Autodesk Inventor part; units mm, degrees
ref_plane "YZ Plane" through (0, 0, 0) normal (1, 0, 0) x (0, 1, 0)
ref_plane "XZ Plane" through (0, 0, 0) normal (0, 1, 0) x (-1, 0, 0)
ref_plane "XY Plane" through (0, 0, 0) normal (0, 0, 1) x (1, 0, 0)
sketch "スケッチ1" plane through (0, 0, 0) normal (0, 0, 1) x (1, 0, 0)
  circle A0 centre (0, 0) radius 60
  dimension "d0" = 120
extrude "押し出し1" add sketch "スケッチ1" along normal blind 3
sketch "スケッチ2" plane through (0, 0, 3) normal (0, 0, 1) x (1, 0, 0)
  circle A0 centre (0, 0) radius 46
  line L0 (0, 0) -> (0, 59.211)
  line L1 (0, 0) -> (-21.8609, 52.777)
  line L2 (0, 0) -> (27.8226, 47.8581)
  point P0 (-17.6034, 42.4985)
  point P1 (-42.4985, 17.6034)
  point P2 (-42.4985, -17.6034)
  point P3 (-17.6034, -42.4985)
  point P4 (17.6034, -42.4985)
  point P5 (42.4985, -17.6034)
  point P6 (42.4985, 17.6034)
  point P7 (17.6034, 42.4985)
  dimension "d4" = 92
  dimension "d5" = 22.5
  dimension "d8" = 360
hole "穴1" at (-17.6034, 42.4985, 3) at (-42.4985, 17.6034, 3) at (-42.4985, -17.6034, 3) at (-17.6034, -42.4985, 3) at (17.6034, -42.4985, 3) at (42.4985, -17.6034, 3) at (42.4985, 17.6034, 3) at (17.6034, 42.4985, 3) direction (0, 0, -1) diameter 3.2 end through all
sketch "スケッチ4" plane through (0, 0, 0) normal (0, 0, -1) x (-1, 0, 0)
  line L0 (0, 0) -> (0, -80.557)
  circle A0 centre (0, 0) radius 60
  line L1 (-60, 0) -> (-60, -190)
  line L2 (60, 0) -> (60, -190)
  line L3 (-60, -190) -> (60, -190)
  line L4 (-60, 0) -> (-43.3772, -190)
  line L5 (10.9847, -144.6101) -> (60, -190)
  line L6 (18.2202, -151.3104) -> (-10.1159, -125.0702)
  line L7 (10, -105.557) -> (10, -25)
  circle A1 centre (0, 0) radius 7
  line L8 (10, -177.6776) -> (0, -177.6776)
  line L9 (0, -177.6776) -> (0, -62.3224)
  line L10 (10, -62.3224) -> (10, -177.6776)
  circle A2 centre (0, -160) radius 4
  circle A3 centre (0, -160) radius 15
  line L11 (27.6237, -152.2466) -> (-9.3418, -192.1645)
  line L12 (15, -160) -> (15, -138.6677)
  line L13 (30, -190) -> (10, -115.4165)
  point P0 (60, 0)
  point P1 (-59.0885, -10.4189)
  point P2 (-60, -25)
  point P3 (60, -25)
  point P4 (10, -59.1608)
  point P5 (10, -143.6982)
  point P6 (0, -134.4378)
  point P7 (0, -60)
  point P8 (0, -60)
  point P9 (10, -120)
  point P10 (10, -171.1803)
  point P11 (11.0058, -170.1918)
  point P12 (10, -171.2779)
  point P13 (21.6159, -158.7342)
  point P14 (-7.3373, -190)
  dimension "d362" = 30
  dimension "d21" = 60
  dimension "d23" = 120
  dimension "d24" = 190
  dimension "d25" = 190
  dimension "d56" = 0
  dimension "d90" = 85
  dimension "d307" = 10
  dimension "d359" = 160
  dimension "d361" = 8
  dimension "d379" = 30
  dimension "d380" = 0
  dimension "d381" = 70
extrude "押し出し3" add sketch "スケッチ4" against normal blind 3 contours L0 A0 L7 L10 L6 L9 | L0 L9 A3 L8 L11 L3 L4 A0 | L6 L10 A3 L9 | L4 L3 L1 A0 | L10 L13 L5 L6 | L6 L5 L12 A3 L10 | A3 L10 L9 A2 | L9 A2 A3 | A3 L10 | A3 L10 L11 L8 L9 | L11 L8 L10 L13 L3 | L5 L13 L11 A3 L12 | A3 L11 L10 | L11 L10 L8
sketch "スケッチ17" plane through (0, 0, 3) normal (0, 0, 1) x (1, 0, 0)
  circle A0 centre (0, 0) radius 30
  dimension "d159" = 60
extrude "押し出し10" cut sketch "スケッチ17" against normal blind 10
sketch "スケッチ20" plane through (0, 0, 3) normal (0, 0, 1) x (1, 0, 0)
  line L0 (-30, -190) -> (60, -190)
  circle A0 centre (0, 0) radius 30
  line L1 (60, -190) -> (60, 0)
  point P0 (0, -160)
  point P1 (15, -190)
  point P2 (-60, -190)
  point P3 (7.3373, -190)
  dimension "d205" = 160
  dimension "d223" = 60
  dimension "d246" = 60
hole "穴8" at (0, -160, 3) direction (0, 0, -1) diameter 8.1 end through all
fillet "フィレット4" radius 10 3 edges at (60, -190, 1.5) (-10, -115.4165, 1.5) (-30, -190, 1.5)
sketch "スケッチ28" plane through (0, 0, 3) normal (0, 0, 1) x (1, 0, 0)
  circle A0 centre (0, 0) radius 60
  circle A1 centre (0, 0) radius 54
  point P0 (0, 54)
  point P1 (-38.1838, 38.1838)
  point P2 (-54, 0)
  point P3 (-38.1838, -38.1838)
  point P4 (0, -54)
  point P5 (38.1838, -38.1838)
  point P6 (54, 0)
  point P7 (38.1838, 38.1838)
  dimension "d309" = 108
  dimension "d308" = 120
  dimension "d312" = 360
hole "穴13" at (-38.1838, -38.1838, 3) at (-54, 0, 3) at (-38.1838, 38.1838, 3) at (0, 54, 3) at (38.1838, 38.1838, 3) at (54, 0, 3) direction (0, 0, -1) diameter 3.2 end through all
sketch "スケッチ29" plane through (0, 0, 3) normal (0, 0, 1) x (1, 0, 0)
  arc A0 (60, 0) -> (-10, -59.1608) centre (0, 0) ccw
  line L0 (-10, -59.1608) -> (0, -59.1608)
  line L1 (0, -59.1608) -> (0, -130)
  line L2 (0, -130) -> (-10, -130)
  line L3 (-10, -130) -> (-10, -59.1608)
  line L4 (60, 0) -> (60, -180)
  line L5 (60, -130) -> (50, -130)
  line L6 (50, -130) -> (50, 10.2883)
  line L7 (50, 10.2883) -> (60, 10.2883)
  line L8 (60, 10.2883) -> (60, -130)
  line L9 (-30, -190) -> (50, -190)
  circle A1 centre (54, 0) radius 1.6
  line L10 (-10, -59.1608) -> (-10, -115.4165)
  point P0 (-35.8579, -190)
  point P1 (54, -40)
  point P2 (-5, -59.1608)
  point P3 (-4, -69.1608)
  point P4 (54, -80)
  point P5 (54, -120)
  point P6 (54, -160)
  point P7 (55, -130)
  point P8 (-5, -130)
  point P9 (-4, -129.1608)
  point P10 (54, -200)
  point P11 (-10, -140)
  point P12 (40, -210)
  point P13 (-40, -210)
  point P14 (-4, -99.1608)
  point P15 (7.3373, -190)
  point P16 (11.7061, -190)
  dimension "d321" = 60
  dimension "d322" = 10
  dimension "d323" = 10
  dimension "d324" = 40
  dimension "d325" = 6
  dimension "d339" = 40
  dimension "d340" = 40
  dimension "d341" = 40
  dimension "d342" = 6
  dimension "d352" = 4
  dimension "d356" = 40
  dimension "d357" = 6
  dimension "d358" = 6
  dimension "d364" = 10
  dimension "d366" = 4
  dimension "d367" = 30
  dimension "d368" = 30
hole "穴14" at (54, -80, 3) at (54, -200, 3) at (54, -160, 3) at (54, -120, 3) at (54, -40, 3) at (-4, -69.1608, 3) at (-4, -99.1608, 3) at (-4, -129.1608, 3) direction (0, 0, -1) diameter 3.2 end through all
fillet "フィレット11" radius 2.5 1 edges at (-10, -59.1608, 1.5)
sketch "スケッチ30" plane through (0, 0, 3) normal (0, 0, 1) x (1, 0, 0)
  point P0 (0, 0)
sketch "スケッチ32" plane through (0, 0, 3) normal (0, 0, 1) x (1, 0, 0)
  circle A0 centre (28, -150) radius 10
  line L0 (60, -180) -> (60, 0)
  point P0 (0, 0)
  dimension "d382" = 20
  dimension "d383" = 150
  dimension "d384" = 32
extrude "押し出し16" cut sketch "スケッチ32" against normal blind 10
equation "\"d25\" = d24"
equation "\"d90\" = d89"
properties part number "RP_Thigh-cover" material "アルミニウム 6061"
Input: part model. Units: mm. Frame: model coordinates. Round coordinates to 2 decimals unless told otherwise and drop trailing zeros. Loops run counter-clockwise (first coordinate to the right, second up) from the corner with the lowest first, then second, coordinate; pieces in that order, holes last. Notation, with made-up numbers: (-8, -26) - (7, -26) arc R25 ccw to (7, -11) - close; hole circle Ø7 at (24, 89). An arc over 180 degrees is marked (long way). One line per item, written item: value. Start each with the question number.
(1) Ray query, line 1 (Y direction, x = 2.5, z = 2.6); line 2 (X direction, y = -39, z = 0.2); line 3 (Y direction, x = 54, z = 1.6). Return the intervals inside material, ascending. Write a range as [from, to].
(2) Section C-C, the plane y = -8.5. Return loops of the section in (x, z), plus the area to 3 significant figures.
(3) Section B-B, the plane z = 0.7. Count the separate pieces of the cut face and the enclosed holes in it, plus the area to 3 significant figures.
(4) Contact query for a flat-ended pin moving along its axis: P1, Ø7.5, axis at x = 0, y = -160, coming from the +Z side. Output: stop coordinate, or through.
(5) Section A-A, the plane y = -150. Return loops of the section in (x, z).
(6) Draft query along X for faces 1 (the cylindrical face through (-39.4, 45.25, 1.48)), 2 (the cylindrical face through (25.83, -159.76, 1.52)), 3 (the flat face through (-18.597, -147.475, 1.479)). Return one class per face: +X half, -X half, draft (parallel to the pull), parting line (faces both ways), or undercut.
(7) Section D-D, the plane x = -33. Return loops of the section in (y, z).
Results below:
1. line 1: [-190, -163.19], [-156.81, -29.9], [29.9, 59.95]
1. line 2: [-45.6, -39.56], [-36.81, 52.75], [55.25, 60]
1. line 3: [-189.17, -161.6], [-158.4, -121.6], [-118.4, -81.6], [-78.4, -41.6], [-38.4, -1.6], [1.6, 26.15]
2. outline: (-59.39, 0) - (-28.77, 0) - (-28.77, 3) - (-59.39, 3) - close; (28.77, 0) - (60, 0) - (60, 3) - (28.77, 3) - close
2. area: 186 mm^2
3. separate pieces: 1
3. enclosed holes: 24
3. area: 18,500 mm^2
4. P1: through
5. outline: (-19.27, 0) - (18, 0) - (18, 3) - (-19.27, 3) - close; (38, 0) - (60, 0) - (60, 3) - (38, 3) - close
6. face 1: parting line
6. face 2: undercut
6. face 3: -X half
7. outline: (-50.11, 0) - (50.11, 0) - (50.11, 3) - (-50.11, 3) - close
